from build123d import *

# Parameters (mm, degrees)
SKETCH_1_W                     = 80
SKETCH_1_H                     = 60
EXTRUDE_1_DEPTH                = 8
HOLE_WIZARD_12_0_12_1_D        = 12
HOLE_WIZARD_10_5_10_5_1_D      = 10.5
HOLE_WIZARD_M3_5_1_D           = 4
HOLE_WIZARD_M3_5_1_CSINK_D     = 7
HOLE_WIZARD_M3_5_1_CSINK_ANGLE = 90
CUT_EXTRUDE_1_DEPTH            = 1
CUT_EXTRUDE_2_REACH            = 95.053
CUT_EXTRUDE_3_REACH            = 94.961
SKETCH_29_W                    = 80
SKETCH_29_H                    = 10


with BuildPart() as part:
    # 草图1 → 凸台-拉伸1 (new body)
    with BuildSketch(Plane(origin=(0, 0, 1), x_dir=(-1, 0, 0), z_dir=(0, 0, -1))):
        with Locations((-40, 16.666666667)):
            Rectangle(SKETCH_1_W, SKETCH_1_H)
    extrude(amount=-EXTRUDE_1_DEPTH)

    # Ø12.0 (12) 直径孔1 (through all)
    with Locations(Plane.XY.offset(9)):
        with Locations((72, 16.666666667), (8, 16.666666667)):
            Hole(HOLE_WIZARD_12_0_12_1_D / 2)

    # Ø10.5 (10.5) 直径孔1 (through all)
    with Locations(Plane(origin=(0, 0, 1), x_dir=(-1, 0, 0), z_dir=(0, 0, -1))):
        with Locations((-40, 16.666666667)):
            Hole(HOLE_WIZARD_10_5_10_5_1_D / 2)

    # M3.5 平头机械螺钉的锥形沉头孔1 (through all)
    with Locations(Plane.XY.offset(9)):
        with Locations((32, 16.666666667), (48, 16.666666667)):
            CounterSinkHole(HOLE_WIZARD_M3_5_1_D / 2, HOLE_WIZARD_M3_5_1_CSINK_D / 2, counter_sink_angle=HOLE_WIZARD_M3_5_1_CSINK_ANGLE)

    # 草图27 → 切除-拉伸1 (cut)
    with BuildSketch(Plane(origin=(0, 0, 1), x_dir=(-1, 0, 0), z_dir=(0, 0, -1))):
        with BuildLine():
            ThreePointArc((-41, 30.666666667), (-40, 29.666666667), (-39, 30.666666667))
            Line((-39, 30.666666667), (-39, 42.666666667))
            Line((-39, 42.666666667), (-21.828427125, 42.666666667))
            Line((-21.828427125, 42.666666667), (-32.414213562, 32.080880229))
            ThreePointArc((-32.414213562, 32.080880229), (-32.414213562, 30.666666667), (-31, 30.666666667))
            Line((-31, 30.666666667), (-19, 42.666666667))
            Line((-19, 42.666666667), (-8, 42.666666667))
            Line((-8, 42.666666667), (-8, 30.666666667))
            ThreePointArc((-8, 30.666666667), (-7, 29.666666667), (-6, 30.666666667))
            Line((-6, 30.666666667), (-6, 42.666666667))
            Line((-6, 42.666666667), (0, 42.666666667))
            Line((0, 42.666666667), (0, 44.666666667))
            Line((0, 44.666666667), (-6, 44.666666667))
            Line((-6, 44.666666667), (-6, 46.666666667))
            Line((-6, 46.666666667), (-8, 46.666666667))
            Line((-8, 46.666666667), (-8, 44.666666667))
            Line((-8, 44.666666667), (-17, 44.666666667))
            Line((-17, 44.666666667), (-15, 46.666666667))
            Line((-15, 46.666666667), (-16.414213562, 48.080880229))
            Line((-16.414213562, 48.080880229), (-19.828427125, 44.666666667))
            Line((-19.828427125, 44.666666667), (-39, 44.666666667))
            Line((-39, 44.666666667), (-39, 46.666666667))
            Line((-39, 46.666666667), (-41, 46.666666667))
            Line((-41, 46.666666667), (-41, 44.666666667))
            Line((-41, 44.666666667), (-60.171572875, 44.666666667))
            Line((-60.171572875, 44.666666667), (-63.585786438, 48.080880229))
            Line((-63.585786438, 48.080880229), (-65, 46.666666667))
            Line((-65, 46.666666667), (-63, 44.666666667))
            Line((-63, 44.666666667), (-72, 44.666666667))
            Line((-72, 44.666666667), (-72, 46.666666667))
            Line((-72, 46.666666667), (-74, 46.666666667))
            Line((-74, 46.666666667), (-74, 44.666666667))
            Line((-74, 44.666666667), (-80, 44.666666667))
            Line((-80, 44.666666667), (-80, 42.666666667))
            Line((-80, 42.666666667), (-74, 42.666666667))
            Line((-74, 42.666666667), (-74, 30.666666667))
            ThreePointArc((-74, 30.666666667), (-73, 29.666666667), (-72, 30.666666667))
            Line((-72, 30.666666667), (-72, 42.666666667))
            Line((-72, 42.666666667), (-61, 42.666666667))
            Line((-61, 42.666666667), (-49, 30.666666667))
            ThreePointArc((-49, 30.666666667), (-47.585786438, 30.666666667), (-47.585786438, 32.080880229))
            Line((-47.585786438, 32.080880229), (-58.171572875, 42.666666667))
            Line((-58.171572875, 42.666666667), (-41, 42.666666667))
            Line((-41, 42.666666667), (-41, 30.666666667))
        make_face()
    extrude(amount=-CUT_EXTRUDE_1_DEPTH, mode=Mode.SUBTRACT)

    # 草图28 → 切除-拉伸2 (cut, up to next)
    with BuildSketch(Plane.ZY, mode=Mode.PRIVATE) as cut_extrude_2_sk1:
        Polygon((9, 46.666666667), (5.8, 46.666666667), (5.8, 45.866666667), (6.6, 45.866666667), (6.6, 45.066666667), (7.4, 45.066666667), (7.4, 44.266666667), (8.2, 44.266666667), (8.2, 43.466666667), (9, 43.466666667), align=None)
    cut_extrude_2_tool1 = extrude(cut_extrude_2_sk1.sketch, amount=-CUT_EXTRUDE_2_REACH, mode=Mode.PRIVATE) & part.part
    add(cut_extrude_2_tool1.solids().sort_by_distance((0, 45.466667, 7.8))[0], mode=Mode.SUBTRACT)

    # 草图29 → 切除-拉伸3 (cut, up to next)
    with BuildSketch(Plane(origin=(0, 0, 1), x_dir=(-1, 0, 0), z_dir=(0, 0, -1)), mode=Mode.PRIVATE) as cut_extrude_3_sk1:
        with Locations((-40, -8.333333333)):
            Rectangle(SKETCH_29_W, SKETCH_29_H)
    cut_extrude_3_tool1 = extrude(cut_extrude_3_sk1.sketch, amount=-CUT_EXTRUDE_3_REACH, mode=Mode.PRIVATE) & part.part
    add(cut_extrude_3_tool1.solids().sort_by_distance((40, -8.333333, 1))[0], mode=Mode.SUBTRACT)


solid = part.part
The listing builds one solid part. Answer for the finished solid, in the listing's coordinates (mm). A direction names the side the tool comes from. Coordinates: 2 decimals unless noted, no trailing zeros. Order: outer loops, then holes, each group sorted by start corner. A loop starts at its lowest first (then second) coordinate and runs counter-clockwise, first axis right, second up.
Q1. A cutting plane is placed at C-C, the plane y = 41. Write down the section's boundary in (x, z).
Q2. For a pull along X with two mould halves and no side action, classify faces 3 (the face through (52, 46, 1)), 4 (the face through (77.994, 16.93, 4.944)) as pulls with the +X half, pulls with the -X half, needs draft (parallel to the pull), parting line crosses it, or undercut.
Q3. Given P1, Ø0.9, axis at x = 41, z = 7.5, coming from the +Y side, flat-ended and moving along its own axis, determine where the tip first touches the part or whether it passes through.
Q4. A cutting plane is placed at A-A, the plane x = 40. Write down the section's boundary in (y, z).
Q5. Which of the six approach directions +Z, -Z, +X, -X, +Y, -Y give full straight-line access (tool end or side, diameter ignored) to faces 1 (the face through (52.805, 37.3, 1.493)), 2 (the face through (29.93, 15.81, 7.74))?
Q6. A cutting plane is placed at D-D, the plane x = 73. Write down the section's boundary in (y, z).
Q7. Consider line 1 (Y direction, x = 40, z = 3.25); line 2 (Y direction, x = 48, z = 4.5); line 3 (X direction, y = 21, z = 3.75). Determine where each line is inside the solid, lowest interval first.
Q8. A cutting plane is placed at B-B, the plane x = 23.5. Write down the section's boundary in (y, z).
Answers follow:
1. outline: (0, 1) - (6, 1) - (6, 2) - (8, 2) - (8, 1) - (20.67, 1) - (20.67, 2) - (23.5, 2) - (23.5, 1) - (39, 1) - (39, 2) - (41, 2) - (41, 1) - (56.5, 1) - (56.5, 2) - (59.33, 2) - (59.33, 1) - (72, 1) - (72, 2) - (74, 2) - (74, 1) - (80, 1) - (80, 9) - (0, 9) - close
2. face 3: needs draft
2. face 4: undercut
3. P1: stops at y = 45.07
4. outline: (-3.33, 1) - (11.42, 1) - (11.42, 9) - (-3.33, 9) - close; (21.92, 1) - (29.67, 1) - (29.67, 2) - (46.67, 2) - (46.67, 5.8) - (45.87, 5.8) - (45.87, 6.6) - (45.07, 6.6) - (45.07, 7.4) - (44.27, 7.4) - (44.27, 8.2) - (43.47, 8.2) - (43.47, 9) - (21.92, 9) - close
5. face 1: -Z
5. face 2: +Z
6. outline: (-3.33, 1) - (10.75, 1) - (10.75, 9) - (-3.33, 9) - close; (22.58, 1) - (29.67, 1) - (29.67, 2) - (46.67, 2) - (46.67, 5.8) - (45.87, 5.8) - (45.87, 6.6) - (45.07, 6.6) - (45.07, 7.4) - (44.27, 7.4) - (44.27, 8.2) - (43.47, 8.2) - (43.47, 9) - (22.58, 9) - close
7. line 1: y = -3.33 to 11.42, 21.92 to 46.67
7. line 2: y = -3.33 to 14.67, 18.67 to 46.67
7. line 3: x = 0 to 3.85, 12.15 to 37.04, 42.96 to 67.85, 76.15 to 80
8. outline: (-3.33, 1) - (38.17, 1) - (38.17, 2) - (41, 2) - (41, 1) - (42.67, 1) - (42.67, 2) - (44.67, 2) - (44.67, 1) - (46.67, 1) - (46.67, 5.8) - (45.87, 5.8) - (45.87, 6.6) - (45.07, 6.6) - (45.07, 7.4) - (44.27, 7.4) - (44.27, 8.2) - (43.47, 8.2) - (43.47, 9) - (-3.33, 9) - close
